Could you check a few things on this model? Use its own coordinates, in mm. Give positions to 0.01 mm unless a question says otherwise; leave off trailing zeros. Loops run counter-clockwise (first coordinate to the right, second up) from the corner with the lowest first, then second, coordinate; pieces in that order, holes last. Notation, with made-up numbers: (-6.5, 58.25) - (1.5, 58.25) arc R35 cw to (1.5, 92.25) - close; hole circle Ø4 at (-28, -38). An arc over 180 degrees is marked (long way). Write each question's results on one line, items separated by ' | '. Start each with the question number.
```python
from build123d import *

# Parameters (mm, degrees)
BOSS_EXTRUDE1_DEPTH = 42
SKETCH2_R           = 3.3
BOSS_EXTRUDE2_DEPTH = 1.8


with BuildPart() as part:
    # Sketch1 → Boss-Extrude1 (new body, symmetric)
    with BuildSketch(Plane(origin=(0, 0, 0), x_dir=(1, 0, 0), z_dir=(0, 1, 0))):
        Polygon((0, 20.075), (0, -20.075), (-2.895827662, -20.075), (-5, 20.075), align=None)
    extrude(amount=BOSS_EXTRUDE1_DEPTH, both=True)

    # Sketch2 → Boss-Extrude2 (add)
    with BuildSketch(Plane(origin=(-3.937100288, 0, 0.206334683), x_dir=(0.052335956, 0, 0.998629535), z_dir=(-0.998629535, 0, 0.052335956))):
        with Locations((-5.109167691, -29.895651858)):
            Circle(SKETCH2_R)
        with Locations((-5.109167691, 29.895651858)):
            Circle(SKETCH2_R)
    extrude(amount=BOSS_EXTRUDE2_DEPTH)


solid = part.part
```
Q1. I want a section at B-B, the plane z = -9.5. List the corners of the cut face in (x, y) for me, then the cut area to 3 significant figures.
Q2. I'm going to push a flat-ended pin straight in: pin 1 Ø2 at (y, z) = (5.5, -1.5) entering from -X. Where does the tip first touch, or does it pass through?
Q3. I need wall thicknesses on L1, parallel to X at y = -16.5, z = 3.5; L2, parallel to X at y = -1.5, z = -2. Which ranges of each line are inside material? Lowest first, please. Write a range as from..to.
Q4. If we mould it in two halves opening along X, with no side actions, what happens to faces 1 (the face through (-5.13, -33.12, -5.56)), 2 (the face through (-6, 29.9, -4.8)), 3 (the face through (0, 1, 0)), 4 (the face through (-1, 1, 20.075))? For each: +X half, -X half, draft (parallel to the pull), parting line (faces both ways), or undercut.
Q5. I want a section at A-A, the plane y = -2. List the corners of the cut face in (x, z) for me (3 decimals), then the cut area to 3 significant figures.
Q6. I want a section at C-C, the plane y = 28.5. List the corners of the cut face in (x, z) for me (3 decimals).
Conclusion:
1) outline: (-4.45, -42) - (0, -42) - (0, 42) - (-4.45, 42) - close | area: 373 mm^2
2) pin 1: x = -4.08
3) L1: -3.76..0 | L2: -4.05..0
4) face 1: undercut | face 2: -X half | face 3: +X half | face 4: draft
5) outline: (-5, -20.075) - (0, -20.075) - (0, 20.075) - (-2.896, 20.075) - close | area: 159 mm^2
6) outline: (-6.159, -7.788) - (-4.361, -7.882) - (-5, -20.075) - (0, -20.075) - (0, 20.075) - (-2.896, 20.075) - (-4.048, -1.91) - (-5.846, -1.815) - close
